Design review of the part built by this model. Coordinates are the model's own, in mm. Coordinates: 2 decimals unless noted, no trailing zeros. Order: outer loops, then holes, each group sorted by start corner. A loop starts at its lowest first (then second) coordinate and runs counter-clockwise, first axis right, second up. Notation, with made-up numbers: M 55.5,78.5 L 59.5,78.5 A29 ccw 59.5,113.5 Z; hole C -20,-11.5 d3. An arc over 180 degrees is marked long. Answer as a JSON object with one key per item and string values.
from build123d import *

# Parameters (mm, degrees)
BOX_W             = 250
BOX_H             = 20
BOX_DEPTH         = 3
CYLINDER_R        = 2.25
CYLINDER_DEPTH    = 3
CYLINDER001_R     = 2.25
CYLINDER001_DEPTH = 3
CYLINDER002_R     = 2.25
CYLINDER002_DEPTH = 3
CYLINDER003_R     = 2.25
CYLINDER003_DEPTH = 3


with BuildPart() as part:
    # Box → Box (join)
    with BuildSketch(Plane.XY):
        with Locations((125, 10)):
            Rectangle(BOX_W, BOX_H)
    extrude(amount=BOX_DEPTH)

    # Cylinder → Cylinder (cut)
    with BuildSketch(Plane(origin=(10, 10, 0), x_dir=(1, 0, 0), z_dir=(0, 0, 1))):
        Circle(CYLINDER_R)
    extrude(amount=CYLINDER_DEPTH, mode=Mode.SUBTRACT)

    # Cylinder001 → Cylinder001 (cut)
    with BuildSketch(Plane(origin=(237, 10, 0), x_dir=(1, 0, 0), z_dir=(0, 0, 1))):
        Circle(CYLINDER001_R)
    extrude(amount=CYLINDER001_DEPTH, mode=Mode.SUBTRACT)

    # Cylinder002 → Cylinder002 (cut)
    with BuildSketch(Plane(origin=(92, 10, 0), x_dir=(1, 0, 0), z_dir=(0, 0, 1))):
        Circle(CYLINDER002_R)
    extrude(amount=CYLINDER002_DEPTH, mode=Mode.SUBTRACT)

    # Cylinder003 → Cylinder003 (cut)
    with BuildSketch(Plane(origin=(158, 10, 0), x_dir=(1, 0, 0), z_dir=(0, 0, 1))):
        Circle(CYLINDER003_R)
    extrude(amount=CYLINDER003_DEPTH, mode=Mode.SUBTRACT)


solid = part.part
1) Insertion check: pin 1 Ø3.5 at (x, y) = (10, 10) entering from -Z. The pin has a flat end and moves straight along its axis. Give the tip position at first contact, or say it passes through.
Taken from the geometry:
{"pin 1": "passes through"}
2) Add section B-B (x = 10). State the section outline as (y, z) points, and give its area (3 significant figures).
Taken from the geometry:
{"outline": "M 0,0 L 7.75,0 L 7.75,3 L 0,3 Z; M 12.25,0 L 20,0 L 20,3 L 12.25,3 Z", "area": "46.5 mm2"}
3) Mouldability with a two-part tool opening along X and no side actions: class faces 1 (the cylindrical face through (94.146, 10.676, 1.479)), 2 (the flat face through (123, 10, 0)) as released by +X, released by -X, zero draft, split by the parting line, or undercut.
Taken from the geometry:
{"face 1": "undercut", "face 2": "zero draft"}
4) To check wall thickness, follow L1, parallel to Y at x = 10, z = 1.35; L2, parallel to X at y = 11, z = 0.7; L3, parallel to X at y = 9.25, z = 2.1. State the ranges of each line that lie inside material, in increasing order.
Taken from the geometry:
{"L1": "y = 0 to 7.75, 12.25 to 20", "L2": "x = 0 to 7.98, 12.02 to 89.98, 94.02 to 155.98, 160.02 to 234.98, 239.02 to 250", "L3": "x = 0 to 7.88, 12.12 to 89.88, 94.12 to 155.88, 160.12 to 234.88, 239.12 to 250"}
5) Add section A-A (y = 10). State the section outline as (x, z) points, and give its area (3 significant figures).
Taken from the geometry:
{"outline": "M 0,0 L 7.75,0 L 7.75,3 L 0,3 Z; M 12.25,0 L 89.75,0 L 89.75,3 L 12.25,3 Z; M 94.25,0 L 155.75,0 L 155.75,3 L 94.25,3 Z; M 160.25,0 L 234.75,0 L 234.75,3 L 160.25,3 Z; M 239.25,0 L 250,0 L 250,3 L 239.25,3 Z", "area": "696 mm2"}
